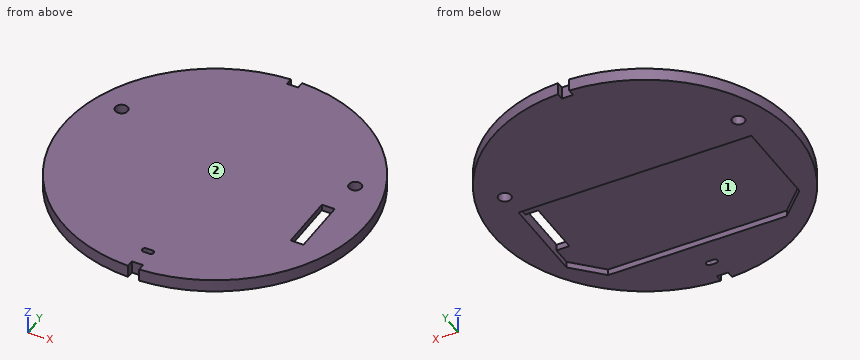
from build123d import *

# Parameters (mm, degrees)
SKETCH1_R           = 1.5
BOSS_EXTRUDE3_DEPTH = 3
BOSS_EXTRUDE4_DEPTH = 1.5


with BuildPart() as part:
    # Sketch1 → Boss-Extrude3 (new body)
    with BuildSketch(Plane.XY):
        with BuildLine():
            Line((-1.35, 36.475025703), (-1.35, 34.723767077))
            ThreePointArc((-1.35, 34.723767077), (0, 34.75), (1.35, 34.723767077))
            Line((1.35, 34.723767077), (1.35, 36.475025703))
            ThreePointArc((1.35, 36.475025703), (36.5, 0), (1.35, -36.475025703))
            Line((1.35, -36.475025703), (1.35, -34.723767077))
            ThreePointArc((1.35, -34.723767077), (0, -34.75), (-1.35, -34.723767077))
            Line((-1.35, -34.723767077), (-1.35, -36.475025703))
            ThreePointArc((-1.35, -36.475025703), (-36.5, 0), (-1.35, 36.475025703))
        make_face()
        with Locations((28.1, 10.5)):
            Circle(SKETCH1_R, mode=Mode.SUBTRACT)
        with Locations((-28.1, 10.5)):
            Circle(SKETCH1_R, mode=Mode.SUBTRACT)
        Polygon((-28, 4.5), (28, 4.5), (28, -17), (21.5, -23.5), (-21.5, -23.5), (-28, -17), align=None, mode=Mode.SUBTRACT)
        with BuildLine():
            Line((-0.75, -29.35), (0.75, -29.35))
            ThreePointArc((0.75, -29.35), (1.4, -30), (0.75, -30.65))
            Line((0.75, -30.65), (-0.75, -30.65))
            ThreePointArc((-0.75, -30.65), (-1.4, -30), (-0.75, -29.35))
        make_face(mode=Mode.SUBTRACT)
    extrude(amount=-BOSS_EXTRUDE3_DEPTH)

    # Sketch1_9 → Boss-Extrude4 (add)
    with BuildSketch(Plane.XY):
        Polygon((28, 4.5), (0, 4.5), (0, -23.5), (21.5, -23.5), (28, -17), (28, -12.5), (24.9, -12.5), (24.9, 1.5), (28, 1.5), align=None)
        Polygon((0, -23.5), (0, 4.5), (-28, 4.5), (-28, -17), (-21.5, -23.5), align=None)
    extrude(amount=-BOSS_EXTRUDE4_DEPTH)


solid = part.part
Read the model definition and answer for the solid it produces. Units are mm, in the model's axes. Face numbers are marked on the shaded views. Round coordinates to 2 decimals unless told otherwise and drop trailing zeros. Loops run counter-clockwise (first coordinate to the right, second up) from the corner with the lowest first, then second, coordinate; pieces in that order, holes last. Notation, with made-up numbers: (-29, 66) - (-13, 66) arc R20 ccw to (-13, 89) - close; hole circle Ø1 at (30.5, 75). An arc over 180 degrees is marked (long way). One line per question, with ' | ' between items. Start each with the question number.
Q1. Section D-D on x = -20.5 is taken. Give the vertices of the cut face in (y, z).
Q2. For a pull along X with two mould halves and no side action, classify the marked faces 1 and 2 as +X half, -X half, draft (parallel to the pull), parting line (faces both ways), or undercut.
Q3. Section A-A on y = 0 is taken. Give the vertices of the cut face in (x, z).
Q4. Flat-ended cylindrical pins translate along their axes: pin 1 (5 mm diameter, centred on x = -28.1, y = 10.5, fed in from -Z); pin 2 (1.2 mm diameter, centred on x = -11, z = -2.5, fed in from -Y); pin 3 (0.8 mm diameter, centred on x = -9, z = -2, fed in from +Y); pin 4 (1.5 mm diameter, centred on y = -7.5, z = -1.5, fed in from -X). Find the tip coordinate at first contact, or state that the pin passes through.
Q5. Section C-C on y = 10.5 is taken. Give the vertices of the cut face in (x, z), plus the area to 3 significant figures.
Q6. Find the intervals of material crossed by L1, parallel to Z at x = -13, y = -9; L2, parallel to Y at x = 28.1, z = -1.8; L3, parallel to Y at x = -12.5, z = -1.8, in increasing order.
Established:
1) outline: (-30.2, -3) - (-23.5, -3) - (-23.5, -1.5) - (4.5, -1.5) - (4.5, -3) - (30.2, -3) - (30.2, 0) - (-30.2, 0) - close
2) face 1: undercut | face 2: draft
3) outline: (-36.5, -3) - (-28, -3) - (-28, -1.5) - (24.9, -1.5) - (24.9, 0) - (-36.5, 0) - close; (28, -3) - (36.5, -3) - (36.5, 0) - (28, 0) - close
4) pin 1: z = -3 | pin 2: y = -34.99 | pin 3: y = 35.47 | pin 4: x = -35.87
5) outline: (-34.96, -3) - (-29.6, -3) - (-29.6, 0) - (-34.96, 0) - close; (-26.6, -3) - (26.6, -3) - (26.6, 0) - (-26.6, 0) - close; (29.6, -3) - (34.96, -3) - (34.96, 0) - (29.6, 0) - close | area: 192 mm²
6) L1: -1.5 to 0 | L2: -23.29 to 9, 12 to 23.29 | L3: -34.29 to -23.5, 4.5 to 34.29
